from build123d import *

# Parameters (mm, degrees)
CYLINDER003_R     = 2
CYLINDER003_DEPTH = 10
CYLINDER002_R     = 2
CYLINDER002_DEPTH = 10
CYLINDER001_R     = 2
CYLINDER001_DEPTH = 10
CYLINDER_R        = 2
CYLINDER_DEPTH    = 10
BOX001_W          = 26
BOX001_H          = 3
BOX001_DEPTH      = 8
BOX002_W          = 9
BOX002_H          = 21
BOX002_DEPTH      = 8
BOX_W             = 50
BOX_H             = 35
BOX_DEPTH         = 8
CYLINDER004_R     = 2
CYLINDER004_DEPTH = 10
CYLINDER005_R     = 2
CYLINDER005_DEPTH = 10
BOX003_W          = 50
BOX003_H          = 35
BOX003_DEPTH      = 3


with BuildPart() as cylinder003:
    # Cylinder003 → Cylinder003 (new body)
    with BuildSketch(Plane(origin=(44, 29, 0), x_dir=(1, 0, 0), z_dir=(0, 0, 1))):
        Circle(CYLINDER003_R)
    extrude(amount=CYLINDER003_DEPTH)


with BuildPart() as cylinder002:
    # Cylinder002 → Cylinder002 (new body)
    with BuildSketch(Plane(origin=(6, 29, 0), x_dir=(1, 0, 0), z_dir=(0, 0, 1))):
        Circle(CYLINDER002_R)
    extrude(amount=CYLINDER002_DEPTH)


with BuildPart() as cylinder001:
    # Cylinder001 → Cylinder001 (new body)
    with BuildSketch(Plane(origin=(44, 6, 0), x_dir=(1, 0, 0), z_dir=(0, 0, 1))):
        Circle(CYLINDER001_R)
    extrude(amount=CYLINDER001_DEPTH)


with BuildPart() as cylinder:
    # Cylinder → Cylinder (new body)
    with BuildSketch(Plane(origin=(6, 6, 0), x_dir=(1, 0, 0), z_dir=(0, 0, 1))):
        Circle(CYLINDER_R)
    extrude(amount=CYLINDER_DEPTH)


with BuildPart() as cube001:
    # Box001 → Box001 (new body)
    with BuildSketch(Plane(origin=(12, 16, 0), x_dir=(1, 0, 0), z_dir=(0, 0, 1))):
        with Locations((13, 1.5)):
            Rectangle(BOX001_W, BOX001_H)
    extrude(amount=BOX001_DEPTH)


with BuildPart() as cube002:
    # Box002 → Box002 (new body)
    with BuildSketch(Plane(origin=(20.5, 7, 0), x_dir=(1, 0, 0), z_dir=(0, 0, 1))):
        with Locations((4.5, 10.5)):
            Rectangle(BOX002_W, BOX002_H)
    extrude(amount=BOX002_DEPTH)


with BuildPart() as cut003:
    # Box → Box (new body)
    with BuildSketch(Plane.XY):
        with Locations((25, 17.5)):
            Rectangle(BOX_W, BOX_H)
    extrude(amount=BOX_DEPTH)

    # Cut: cut Cube002
    add(cube002.part, mode=Mode.SUBTRACT)

    # Cut003: cut Cube001
    add(cube001.part, mode=Mode.SUBTRACT)


with BuildPart() as cylinder004:
    # Cylinder004 → Cylinder004 (new body)
    with BuildSketch(Plane(origin=(25, 22.755, 0), x_dir=(1, 0, 0), z_dir=(0, 0, 1))):
        Circle(CYLINDER004_R)
    extrude(amount=CYLINDER004_DEPTH)


with BuildPart() as cylinder005:
    # Cylinder005 → Cylinder005 (new body)
    with BuildSketch(Plane(origin=(25, 12.25, 0), x_dir=(1, 0, 0), z_dir=(0, 0, 1))):
        Circle(CYLINDER005_R)
    extrude(amount=CYLINDER005_DEPTH)


with BuildPart() as cut007:
    # Box003 → Box003 (new body)
    with BuildSketch(Plane.XY):
        with Locations((25, 17.5)):
            Rectangle(BOX003_W, BOX003_H)
    extrude(amount=BOX003_DEPTH)

    # Cut001: cut Cylinder005
    add(cylinder005.part, mode=Mode.SUBTRACT)

    # Cut002: cut Cylinder004
    add(cylinder004.part, mode=Mode.SUBTRACT)

    # Fusion: union Cut003
    add(cut003.part)

    # Cut004: cut Cylinder
    add(cylinder.part, mode=Mode.SUBTRACT)

    # Cut005: cut Cylinder001
    add(cylinder001.part, mode=Mode.SUBTRACT)

    # Cut006: cut Cylinder002
    add(cylinder002.part, mode=Mode.SUBTRACT)

    # Cut007: cut Cylinder003
    add(cylinder003.part, mode=Mode.SUBTRACT)


solid = cut007.part
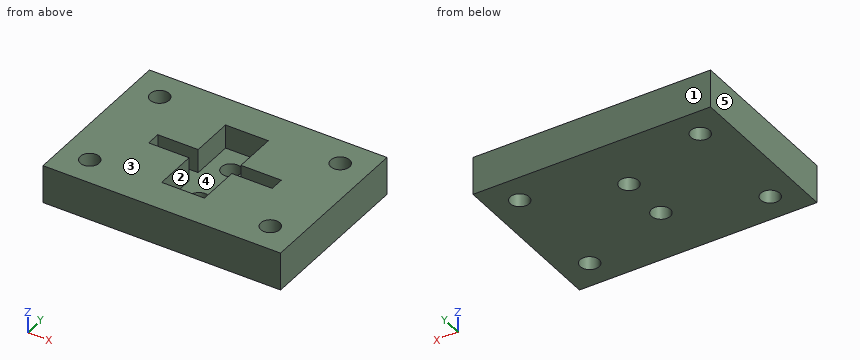
Design review of the part built by this model. Coordinates are the model's own, in mm. Face numbers are marked on the shaded views. A direction names the side the tool comes from. Give positions to 0.01 mm unless a question says otherwise; leave off trailing zeros. Order: outer loops, then holes, each group sorted by start corner. A loop starts at its lowest first (then second) coordinate and runs counter-clockwise, first axis right, second up. Notation, with made-up numbers: (73.25, 13) - (125.25, 13) arc R24 cw to (125.25, 30) - close; hole circle Ø3 at (17, 2). An arc over 180 degrees is marked (long way). Write item = value, one per line. Start each with the question number.
Q1. We need section B-B on x = 25. State the section outline as (y, z) points (3 decimals), plus the area to 3 significant figures.
Q2. Clearance check with a flat-ended pin moving along its axis: pin 1 Ø5 at (x, y) = (25, 22.755) entering from +Z. State where the tip first meets the part, or that it passes through.
Q3. We need section C-C on z = 3.5. State the section outline as (x, y) points.
Q4. Mouldability with a two-part tool opening along X and no side actions: class the marked faces 3, 4 and 5 as released by +X, released by -X, zero draft, split by the parting line, or undercut.
Q5. To check wall thickness, follow L1, parallel to Y at x = 25, z = 1.4 (3 decimals); L2, parallel to X at y = 29, z = 6; L3, parallel to Y at x = 6, z = 6. State the ranges of each line that lie inside material, in increasing order. Write a range as from..to.
Q6. We need section A-A on y = 6. State the section outline as (x, z) points, plus the area to 3 significant figures.
Q7. We need section D-D on y = 12.25. State the section outline as (x, z) points.
Q8. Tool access review of the marked faces 1 and 2: name each direction out of +Z, -Z, +X, -X, +Y, -Y from which nothing blocks a thin tool from reaching the whole face with its end or side.
Working result:
q1.outline = (0, 0) - (10.25, 0) - (10.25, 3) - (7, 3) - (7, 8) - (0, 8) - close; (14.25, 0) - (20.755, 0) - (20.755, 3) - (14.25, 3) - close; (24.755, 0) - (35, 0) - (35, 8) - (28, 8) - (28, 3) - (24.755, 3) - close
q1.area = 151 mm²
q2.pin_1 = 3
q3.outline = (0, 0) - (50, 0) - (50, 35) - (0, 35) - close; hole circle Ø4 at (6, 6); hole circle Ø4 at (6, 29); hole (12, 16) - (20.5, 16) - (20.5, 7) - (29.5, 7) - (29.5, 16) - (38, 16) - (38, 19) - (29.5, 19) - (29.5, 28) - (20.5, 28) - (20.5, 19) - (12, 19) - close; hole circle Ø4 at (44, 6); hole circle Ø4 at (44, 29)
q4.face_3 = zero draft
q4.face_4 = undercut
q4.face_5 = released by -X
q5.L1 = 0..10.25, 14.25..20.755, 24.755..35
q5.L2 = 0..4, 8..42, 46..50
q5.L3 = 0..4, 8..27, 31..35
q6.outline = (0, 0) - (4, 0) - (4, 8) - (0, 8) - close; (8, 0) - (42, 0) - (42, 8) - (8, 8) - close; (46, 0) - (50, 0) - (50, 8) - (46, 8) - close
q6.area = 336 mm²
q7.outline = (0, 0) - (23, 0) - (23, 3) - (20.5, 3) - (20.5, 8) - (0, 8) - close; (27, 0) - (50, 0) - (50, 8) - (29.5, 8) - (29.5, 3) - (27, 3) - close
q8.face_1 = +Z, -Z, +X, -X, +Y
q8.face_2 = +Z
